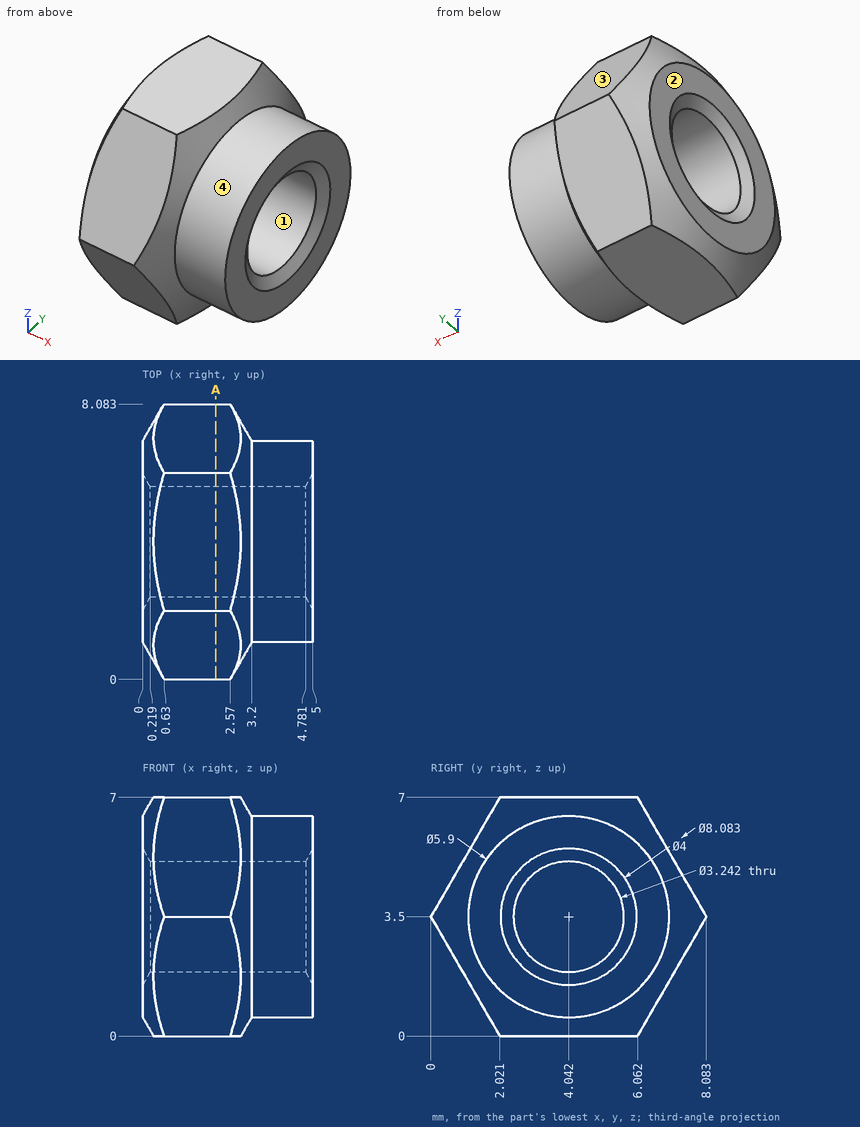
The drawing under review shows one solid part. Ordinate dimensions are in mm from its lowest x, y, z. Coordinates: 2 decimals unless noted, no trailing zeros. Order: outer loops, then holes, each group sorted by start corner. A loop starts at its lowest first (then second) coordinate and runs counter-clockwise, first axis right, second up. Notation, with made-up numbers: (47.5, 48) -> (67.5, 48) arc R20 cw to (67.5, 54) -> close; hole circle Ø9 at (79.25, 15). An arc over 180 degrees is marked (long way). Answer in a Markdown table with one row per item. Add a question column.
Item 1: To check wall thickness, follow probe 1 along Y at (x, z) = (3.25, 3.5); probe 2 along Z at (x, y) = (4.55, 4); probe 3 along Y at (x, z) = (2.8, 3.5) (1 decimal). State the ranges of each line that lie inside material, in increasing order.
Item 2: Clearance check with a flat-ended pin moving along its axis: pin 1 (1.5 mm diameter, centred on x = 4.5, y = 4, fed in from -Z). State where the tip first meets the part, or that it passes through.
Item 3: We need section A-A on x = 2.15. Write out the cut boundary in (y, z).
Item 4: Mouldability with a two-part tool opening along Y and no side actions: class the marked faces 1, 2, 3 and 4 as +Y half, -Y half, draft (parallel to the pull), parting line (faces both ways), or undercut.
Final values:
| question | item | result |
|---|---|---|
| 1 | probe 1 | y = 1.09 to 2.42, 5.66 to 6.99 |
| 1 | probe 2 | z = 0.55 to 1.88, 5.12 to 6.45 |
| 1 | probe 3 | y = 0.4 to 2.4, 5.7 to 7.7 |
| 2 | pin 1 | stops at z = 0.55 |
| 3 | outline | (0, 3.5) -> (2.02, 0) -> (6.06, 0) -> (8.08, 3.5) -> (6.06, 7) -> (2.02, 7) -> close; hole circle Ø3.24 at (4.04, 3.5) |
| 4 | face 1 | undercut |
| 4 | face 2 | draft |
| 4 | face 3 | +Y half |
| 4 | face 4 | parting line |
